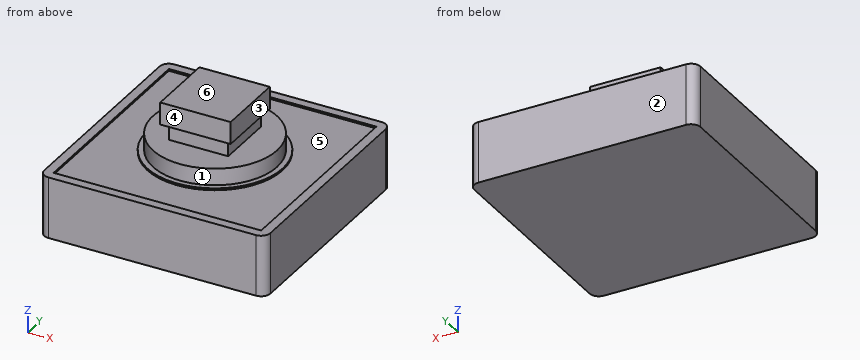
Autodesk Inventor part; units mm, degrees
ref_plane "YZ Plane" through (0, 0, 0) normal (1, 0, 0) x (0, 1, 0)
ref_plane "XZ Plane" through (0, 0, 0) normal (0, 1, 0) x (-1, 0, 0)
ref_plane "XY Plane" through (0, 0, 0) normal (0, 0, 1) x (1, 0, 0)
sketch "스케치1" plane through (0, 0, 0) normal (0, 0, 1) x (1, 0, 0)
  line L0 (-6.1, 6.1) -> (6.1, 6.1)
  line L1 (6.1, 6.1) -> (6.1, -6.1)
  line L2 (6.1, -6.1) -> (-6.1, -6.1)
  line L3 (-6.1, -6.1) -> (-6.1, 6.1)
  line L4 (-6.1, 6.1) -> (6.1, -6.1) construction
  line L5 (6.1, 6.1) -> (-6.1, -6.1) construction
  circle A0 centre (0, 0) radius 3.35
  line L6 (-1.6, 1.6) -> (1.6, 1.6)
  line L7 (1.6, 1.6) -> (1.6, -1.6)
  line L8 (1.6, -1.6) -> (-1.6, -1.6)
  line L9 (-1.6, -1.6) -> (-1.6, 1.6)
  line L10 (-1.6, 1.6) -> (1.6, -1.6) construction
  line L11 (1.6, 1.6) -> (-1.6, -1.6) construction
  line L12 (-1.9, 1.9) -> (1.9, 1.9)
  line L13 (1.9, 1.9) -> (1.9, -1.9)
  line L14 (1.9, -1.9) -> (-1.9, -1.9)
  line L15 (-1.9, -1.9) -> (-1.9, 1.9)
  line L16 (-1.9, 1.9) -> (1.9, -1.9) construction
  line L17 (1.9, 1.9) -> (-1.9, -1.9) construction
  point P0 (0, 0)
  dimension "d0" = 12.2
  dimension "d1" = 12.2
  dimension "d2" = 6.7
  dimension "d3" = 3.2
  dimension "d4" = 3.2
  dimension "d5" = 3.8
  dimension "d6" = 3.8
extrude "돌출1" add sketch "스케치1" against normal blind 3.3 contours L0 L1 L2 L3 | A0 | L6 L7 L8 L9 | L12 L13 L14 L15
extrude "돌출2" add sketch "스케치1" along normal blind 0.9 contours A0 | L6 L7 L8 L9 | L12 L13 L14 L15
extrude "돌출3" add sketch "스케치1" along normal blind 3 contours L6 L7 L8 L9 | L12 L13 L14 L15
sketch "스케치2" plane through (0, 0, 0.9) normal (0, 0, 1) x (1, 0, 0)
  line L0 (-1.6, -1.6) -> (1.6, -1.6)
  line L1 (1.6, -1.6) -> (1.6, 1.6)
  line L2 (1.6, 1.6) -> (-1.6, 1.6)
  line L3 (-1.6, 1.6) -> (-1.6, -1.6)
  line L4 (-1.6, -1.6) -> (1.6, 1.6) construction
  line L5 (1.6, -1.6) -> (-1.6, 1.6) construction
  line L6 (-1.9, -1.9) -> (1.9, -1.9)
  line L7 (1.9, -1.9) -> (1.9, 1.9)
  line L8 (1.9, 1.9) -> (-1.9, 1.9)
  line L9 (-1.9, 1.9) -> (-1.9, -1.9)
  point P0 (0, 0)
  dimension "d13" = 3.2
  dimension "d14" = 3.2
extrude "돌출4" cut sketch "스케치2" along normal blind 0.9
fillet "모깎기1" radius 0.5 4 edges at (6.1, 6.1, -1.65) (6.1, -6.1, -1.65) (-6.1, -6.1, -1.65) (-6.1, 6.1, -1.65)
sketch "스케치3" plane through (0, 0, 0) normal (0, 0, 1) x (1, 0, 0)
  circle A0 centre (0, 0) radius 3.35
  arc A1 (-5.6, 6.1) -> (-6.1, 5.6) centre (-5.6, 5.6) ccw
  line L0 (-6.1, 5.6) -> (-6.1, -5.6)
  arc A2 (-6.1, -5.6) -> (-5.6, -6.1) centre (-5.6, -5.6) ccw
  line L1 (-5.6, -6.1) -> (5.6, -6.1)
  arc A3 (5.6, -6.1) -> (6.1, -5.6) centre (5.6, -5.6) ccw
  line L2 (6.1, -5.6) -> (6.1, 5.6)
  arc A4 (6.1, 5.6) -> (5.6, 6.1) centre (5.6, 5.6) ccw
  line L3 (5.6, 6.1) -> (-5.6, 6.1)
  line L4 (-5.6, 5.6) -> (-5.6, -5.6)
  line L5 (-5.6, -5.6) -> (5.6, -5.6)
  line L6 (5.6, -5.6) -> (5.6, 5.6)
  line L7 (5.6, 5.6) -> (-5.6, 5.6)
  circle A5 centre (0, 0) radius 3.65
  point P0 (0, 0)
  dimension "d18" = 0.5
  dimension "d19" = 0.3
extrude "돌출5" cut sketch "스케치3" against normal blind 0.1 contours L7 L6 L5 L4
properties part number "텍트 스위치"
Work out the finished part from the listing and answer in its coordinate system (mm). Face numbers are marked on the shaded views. A direction names the side the tool comes from. Round coordinates to 2 decimals unless told otherwise and drop trailing zeros. Write each loop counter-clockwise with the first axis right and the second up, starting at its lowest first coordinate (ties: lowest second). Pieces come first, ordered by that corner, then holes.
1) A cutting plane is placed at D-D (z = 1.25). Give the vertices of the cut face in (x, y).
2) A cutting plane is placed at C-C (y = -1.75). Give the vertices of the cut face in (x, z), plus the area to 3 significant figures.
3) A cutting plane is placed at A-A (y = 5.25). Give the vertices of the cut face in (x, z).
4) Given pin 1 Ø3 at (x, z) = (-2.5, 1) entering from -Y; pin 2 Ø1 at (y, z) = (-0.5, 1) entering from +X; pin 3 Ø1 at (x, z) = (-0.5, 1.5) entering from +Y; pin 4 Ø1 at (y, z) = (0.5, 2.5) entering from +X, each flat-ended and moving along its own axis, determine where each tip first touches the part or whether it passes through.
5) A tool of negligible diameter and unlimited length cuts with its end or side. For the marked faces 1, 2 and 3, from which of +Z, -Z, +X, -X, +Y, -Y can it reach the whole face along a straight path? Write none if from no direction.
6) Straight lines are drawn through the part: line 1 (X direction, y = -0.75, z = 2.75); line 2 (Z direction, x = 1, y = -1.75); line 3 (Z direction, x = -4.5, y = 5.75). For each, find the intervals that lie inside material, in ascending order.
7) The mould has two halves that part along Y. Classify the marked faces 4, 5 and 6: pulls with the +Y half, pulls with the -Y half, needs draft (parallel to the pull), parting line crosses it, or undercut.
Completed:
1. outline: (-1.6, -1.6) - (1.6, -1.6) - (1.6, 1.6) - (-1.6, 1.6) - close
2. outline: (-6.1, -3.3) - (6.1, -3.3) - (6.1, 0) - (5.6, 0) - (5.6, -0.1) - (3.2, -0.1) - (3.2, 0) - (2.86, 0) - (2.86, 0.9) - (-2.86, 0.9) - (-2.86, 0) - (-3.2, 0) - (-3.2, -0.1) - (-5.6, -0.1) - (-5.6, 0) - (-6.1, 0) - close; (-1.9, 1.8) - (1.9, 1.8) - (1.9, 3) - (-1.9, 3) - close
2. area: 49.5 mm2
3. outline: (-6.1, -3.3) - (6.1, -3.3) - (6.1, 0) - (5.6, 0) - (5.6, -0.1) - (-5.6, -0.1) - (-5.6, 0) - (-6.1, 0) - close
4. pin 1: stops at y = -6.1
4. pin 2: stops at x = 3.35
4. pin 3: stops at y = 1.9
4. pin 4: stops at x = 1.9
5. face 1: +Z
5. face 2: +Z, -Z, +X, -X, +Y
5. face 3: +Z, +X, +Y, -Y
6. line 1: x = -1.9 to 1.9
6. line 2: z = -3.3 to 0.9, 1.8 to 3
6. line 3: z = -3.3 to 0
7. face 4: pulls with the -Y half
7. face 5: undercut
7. face 6: needs draft
